Autodesk Inventor part; units mm, degrees
ref_plane "YZ Plane" through (0, 0, 0) normal (1, 0, 0) x (0, 1, 0)
ref_plane "XZ Plane" through (0, 0, 0) normal (0, 1, 0) x (-1, 0, 0)
ref_plane "XY Plane" through (0, 0, 0) normal (0, 0, 1) x (1, 0, 0)
sketch "Sketch1" plane through (0, 0, 0) normal (0, 0, 1) x (1, 0, 0)
  line L0 (0, 0) -> (190.5, 0)
  line L1 (190.5, 0) -> (190.5, 150)
  line L2 (190.5, 150) -> (0, 150)
  line L3 (0, 150) -> (0, 0)
  dimension "d0" = 150
  dimension "d1" = 190.5
extrude "Extrusion1" add sketch "Sketch1" along normal blind 8.89
sketch "Sketch2" plane through (0, 0, 8.89) normal (0, 0, 1) x (1, 0, 0)
  line L0 (45.25, 15) -> (145.25, 15) construction
  line L1 (145.25, 15) -> (145.25, 65) construction
  line L2 (145.25, 65) -> (45.25, 65) construction
  line L3 (45.25, 65) -> (45.25, 15) construction
  line L4 (190.5, 150) -> (0, 150) construction
  line L5 (190.5, 0) -> (190.5, 150) construction
  circle A0 centre (45.25, 65) radius 4
  circle A1 centre (145.25, 65) radius 4
  circle A2 centre (45.25, 15) radius 4
  circle A3 centre (145.25, 15) radius 4
  line L6 (0, 0) -> (190.5, 0)
  point P0 (95.25, 65)
  point P1 (95.25, 150)
  point P2 (145.25, 40)
  dimension "d4" = 100
  dimension "d5" = 50
  dimension "d6" = 8
  dimension "d23" = 15
extrude "Extrusion2" cut sketch "Sketch2" against normal up to surface (8.89 mm away)
sketch "Sketch3" plane through (0, 0, 8.89) normal (0, 0, 1) x (1, 0, 0)
  line L0 (7.75, 90) -> (62.75, 90) construction
  line L1 (62.75, 90) -> (62.75, 130) construction
  line L2 (62.75, 130) -> (7.75, 130) construction
  line L3 (7.75, 130) -> (7.75, 90) construction
  circle A0 centre (7.75, 130) radius 2.5
  circle A1 centre (62.75, 130) radius 2.5
  circle A2 centre (7.75, 90) radius 2.5
  circle A3 centre (62.75, 90) radius 2.5
  line L4 (190.5, 150) -> (0, 150) construction
  line L5 (95.25, 150) -> (95.25, 0)
  line L6 (0, 0) -> (190.5, 0) construction
  circle A4 centre (182.75, 130) radius 2.5
  circle A5 centre (127.75, 130) radius 2.5
  circle A6 centre (182.75, 90) radius 2.5
  circle A7 centre (127.75, 90) radius 2.5
  point P0 (62.75, 110)
  point P1 (35.25, 130)
  dimension "d9" = 5
  dimension "d10" = 55
  dimension "d11" = 40
  dimension "d12" = 60
  dimension "d22" = 20
extrude "Extrusion3" cut sketch "Sketch3" against normal up to surface (8.89 mm away)
sketch "Sketch4" plane through (0, 0, 8.89) normal (0, 0, 1) x (1, 0, 0)
  line L0 (77.75, 120) -> (112.75, 120) construction
  line L1 (112.75, 120) -> (112.75, 144) construction
  line L2 (112.75, 144) -> (77.75, 144) construction
  line L3 (77.75, 144) -> (77.75, 120) construction
  circle A0 centre (112.75, 120) radius 2.5
  circle A1 centre (112.75, 144) radius 2.5
  circle A2 centre (77.75, 144) radius 2.5
  circle A3 centre (77.75, 120) radius 2.5
  line L4 (190.5, 150) -> (0, 150) construction
  line L5 (190.5, 0) -> (190.5, 150) construction
  point P0 (0, 0)
  point P1 (95.25, 120)
  point P2 (95.25, 150)
  point P3 (190.5, 75)
  point P4 (112.75, 132)
  dimension "d15" = 5
  dimension "d16" = 35
  dimension "d17" = 24
  dimension "d18" = 6
extrude "Extrusion4" cut sketch "Sketch4" against normal up to surface (8.89 mm away)
properties part number "Spindle_Mounting_Plate"
Work out the finished part from the listing and answer in its coordinate system (mm). Coordinates: 2 decimals unless noted, no trailing zeros. Write each loop counter-clockwise with the first axis right and the second up, starting at its lowest first coordinate (ties: lowest second). Pieces come first, ordered by that corner, then holes.
Q1. A cutting plane is placed at B-B, the plane y = 65. Give the vertices of the cut face in (x, z).
Q2. Find the intervals of material crossed by line 1 (X direction, y = 130, z = 6.75); line 2 (X direction, y = 144, z = 5); line 3 (Y direction, x = 182.75, z = 4), in increasing order.
Q3. A cutting plane is placed at A-A, the plane x = 127.75. Give the vertices of the cut face in (y, z).
Q4. This flat-tipped pin is pushed along its axis until it touches: pin 1 Ø7 at (x, y) = (45.25, 15) entering from +Z. Where does it stop, or does it pass through?
Q5. A cutting plane is placed at D-D, the plane y = 90. Give the vertices of the cut face in (x, z), then the cut area to 3 significant figures.
Q6. Determine the mould class of faces 1 (the face through (190.5, 74, 4)), 2 (the face through (97, 150, 4)), 3 (the face through (185.135, 90.751, 4.507)), 4 (the face through (62.42, 92.48, 4.51)) for opening direction X: released by +X, released by -X, zero draft, split by the parting line, or undercut.
Q7. A cutting plane is placed at C-C, the plane z = 6. State how many separate pieces and enclosed holes the cut face has, then the cut area to 3 significant figures.
Findings below:
1. outline: (0, 0) - (41.25, 0) - (41.25, 8.89) - (0, 8.89) - close; (49.25, 0) - (141.25, 0) - (141.25, 8.89) - (49.25, 8.89) - close; (149.25, 0) - (190.5, 0) - (190.5, 8.89) - (149.25, 8.89) - close
2. line 1: x = 0 to 5.25, 10.25 to 60.25, 65.25 to 125.25, 130.25 to 180.25, 185.25 to 190.5
2. line 2: x = 0 to 75.25, 80.25 to 110.25, 115.25 to 190.5
2. line 3: y = 0 to 87.5, 92.5 to 127.5, 132.5 to 150
3. outline: (0, 0) - (87.5, 0) - (87.5, 8.89) - (0, 8.89) - close; (92.5, 0) - (127.5, 0) - (127.5, 8.89) - (92.5, 8.89) - close; (132.5, 0) - (150, 0) - (150, 8.89) - (132.5, 8.89) - close
4. pin 1: passes through
5. outline: (0, 0) - (5.25, 0) - (5.25, 8.89) - (0, 8.89) - close; (10.25, 0) - (60.25, 0) - (60.25, 8.89) - (10.25, 8.89) - close; (65.25, 0) - (125.25, 0) - (125.25, 8.89) - (65.25, 8.89) - close; (130.25, 0) - (180.25, 0) - (180.25, 8.89) - (130.25, 8.89) - close; (185.25, 0) - (190.5, 0) - (190.5, 8.89) - (185.25, 8.89) - close
5. area: 1,520 mm2
6. face 1: released by +X
6. face 2: zero draft
6. face 3: undercut
6. face 4: undercut
7. separate pieces: 1
7. enclosed holes: 16
7. area: 28,100 mm2
